Verification items for this drawing (mm, ordinates from the low corner). A direction names the side the tool comes from. Give positions to 0.01 mm unless a question says otherwise; leave off trailing zeros. Loops run counter-clockwise (first coordinate to the right, second up) from the corner with the lowest first, then second, coordinate; pieces in that order, holes last. Notation, with made-up numbers: M -40,-19 L 11,-19 A33 cw 11,12 Z; hole C 17,2 d2. An arc over 180 degrees is marked long. Put each result on its own line as item: value. Start each with the question number.
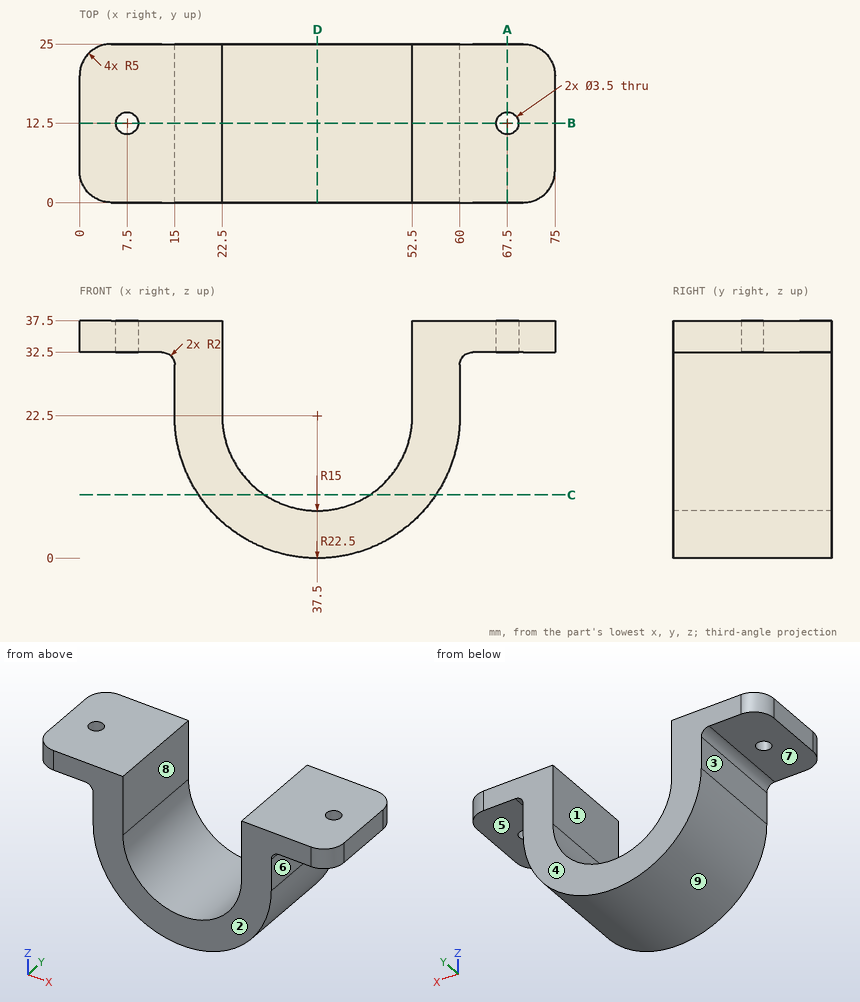
Q1. Cross-section at D-D, the plane x = 37.5. Record the boundary of the cut face in (y, z), then the cut area to 4 significant figures.
Q2. Cross-section at B-B, the plane y = 12.5. Record the boundary of the cut face in (x, z), then the cut area to 3 significant figures.
Q3. Release check for a two-part mould opening along X. For the marked faces 6, 7, 8 and 9 record: pulls with the +X half, pulls with the -X half, needs draft (parallel to the pull), parting line crosses it, or undercut.
Q4. Cross-section at C-C, the plane z = 10. Record the boundary of the cut face in (x, y), then the cut area to 3 significant figures.
Q5. Scan lines: L1, parallel to Y at x = 67.5, z = 35.9; L2, parallel to X at y = 23.75, z = 29.5; L3, parallel to X at y = 5, z = 35.5. Record each from-to range of solid material in increasing order.
Q6. Go/stop test with flat-tipped pins: pin 1 (2.5 mm diameter, centred on y = 15, z = 28, fed in from +X); pin 2 (4.5 mm diameter, centred on y = 12.5, z = 29, fed in from -X); pin 3 (6.5 mm diameter, centred on x = 6.5, y = 13.5, fed in from -Z); pin 4 (3 mm diameter, centred on x = 7.5, y = 12.5, fed in from -Z). Record where each tip stops, or that it passes through.
Q7. Set-up check for the marked faces 1, 2, 3, 4 and 5: record each of +Z, -Z, +X, -X, +Y, -Y from which the full face is reachable in a straight line by a thin tool's end or side.
Q8. Cross-section at A-A, the plane x = 67.5. Record the boundary of the cut face in (y, z), then the cut area to 4 significant figures.
Ans:
1. outline: M 0,0 L 25,0 L 25,7.5 L 0,7.5 Z
1. area: 187.5 mm^2
2. outline: M 0,32.5 L 5.75,32.5 L 5.75,37.5 L 0,37.5 Z; M 9.25,32.5 L 13,32.5 A2 cw 15,30.5 L 15,22.5 A22.5 ccw 60,22.5 L 60,30.5 A2 cw 62,32.5 L 65.75,32.5 L 65.75,37.5 L 52.5,37.5 L 52.5,22.5 A15 cw 22.5,22.5 L 22.5,37.5 L 9.25,37.5 Z; M 69.25,32.5 L 75,32.5 L 75,37.5 L 69.25,37.5 Z
2. area: 784 mm^2
3. face 6: pulls with the +X half
3. face 7: needs draft
3. face 8: undercut
3. face 9: parting line crosses it
4. outline: M 18.79,0 L 29.21,0 L 29.21,25 L 18.79,25 Z; M 45.79,0 L 56.21,0 L 56.21,25 L 45.79,25 Z
4. area: 521 mm^2
5. L1: y = 0 to 10.75, 14.25 to 25
5. L2: x = 15 to 22.5, 52.5 to 60
5. L3: x = 0 to 22.5, 52.5 to 75
6. pin 1: stops at x = 60
6. pin 2: stops at x = 14.85
6. pin 3: stops at z = 32.5
6. pin 4: passes through
7. face 1: +Z, +Y, -Y
7. face 2: +Z, -Z, +X, -X, -Y
7. face 3: -Z, -X, +Y, -Y
7. face 4: +Z, -Z, +X, -X, +Y
7. face 5: -Z, +X, +Y, -Y
8. outline: M 0,32.5 L 10.75,32.5 L 10.75,37.5 L 0,37.5 Z; M 14.25,32.5 L 25,32.5 L 25,37.5 L 14.25,37.5 Z
8. area: 107.5 mm^2
